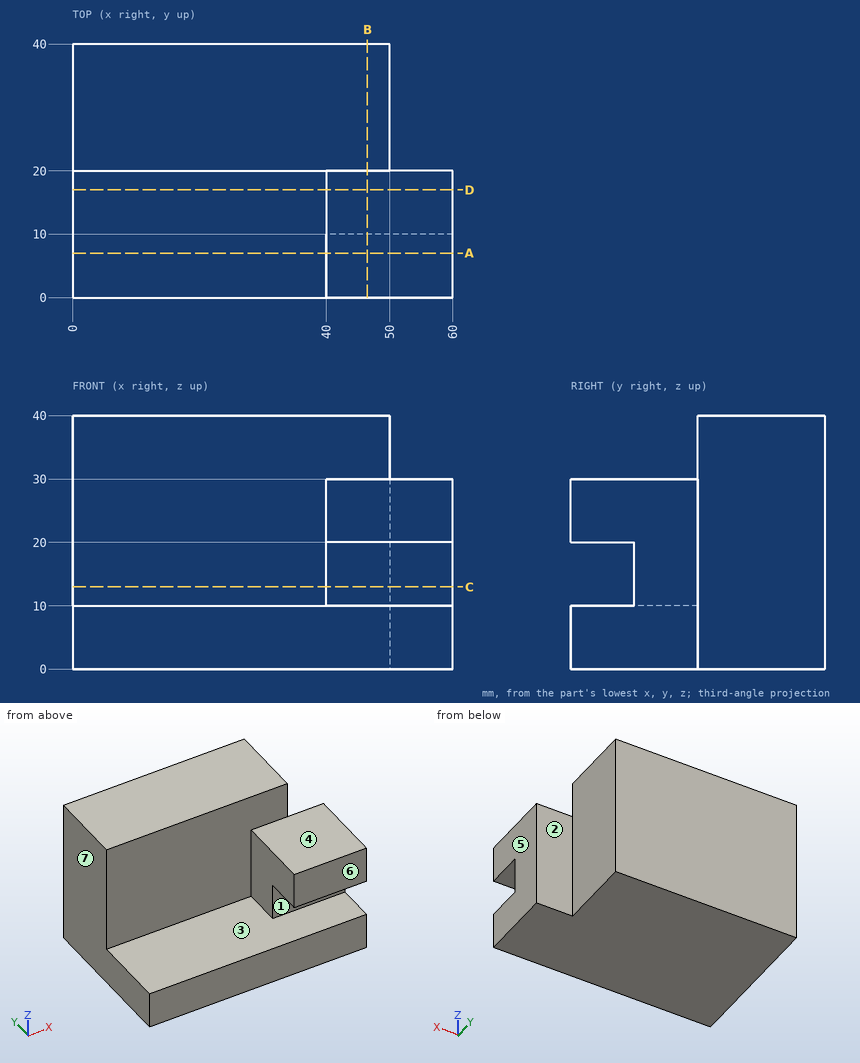
Drawing for the job (mm, zero at the part's lowest x, y, z). A direction names the side the tool comes from. Round coordinates to 2 decimals unless told otherwise and drop trailing zeros. Order: outer loops, then holes, each group sorted by start corner. A loop starts at its lowest first (then second) coordinate and runs counter-clockwise, first axis right, second up.
Item 1: Saw through at D-D on y = 17. Write the cut outline in (x, z), then the cut area to 3 significant figures.
Item 2: Saw through at B-B on x = 46.5. Write the cut outline in (y, z), then the cut area to 3 significant figures.
Item 3: Mould opens along X. For the marked faces 5, 6 and 7 say: pulls with the +X half, pulls with the -X half, needs draft (parallel to the pull), parting line crosses it, or undercut.
Item 4: Saw through at C-C on z = 13. Write the cut outline in (x, y), then the cut area to 3 significant figures.
Item 5: Pin check, flat tips, straight feed: pin 1 (5 mm diameter, centred on x = 47.5, y = 4.5, fed in from -Z); pin 2 (3 mm diameter, centred on x = 54, z = 18.5, fed in from +Y); pin 3 (6 mm diameter, centred on x = 15.5, y = 10, fed in from +Z); pin 4 (10 mm diameter, centred on y = 29, z = 17, fed in from +X). Stop position of each tip, or through.
Item 6: Saw through at A-A on y = 7. Write the cut outline in (x, z), then the cut area to 3 significant figures.
Item 7: Probe line 1 along Z through (x, y) = (16.5, 10.5); line 2 along X through (y, z) = (8, 22); line 3 along Y through (x, z) = (15.5, 14.5). List the from-to ranges inside material, lowest first.
Item 8: Tool access for the marked faces 1, 2, 3 and 4: list every direction of +Z, -Z, +X, -X, +Y, -Y with a clear straight run to the whole face (end or side of a thin tool).
Reported:
1. outline: (0, 0) - (60, 0) - (60, 30) - (40, 30) - (40, 10) - (0, 10) - close
1. area: 1,000 mm2
2. outline: (0, 0) - (40, 0) - (40, 40) - (20, 40) - (20, 30) - (0, 30) - (0, 20) - (10, 20) - (10, 10) - (0, 10) - close
2. area: 1,300 mm2
3. face 5: pulls with the +X half
3. face 6: needs draft
3. face 7: pulls with the -X half
4. outline: (0, 20) - (40, 20) - (40, 10) - (60, 10) - (60, 20) - (50, 20) - (50, 40) - (0, 40) - close
4. area: 1,200 mm2
5. pin 1: stops at z = 0
5. pin 2: stops at y = 20
5. pin 3: stops at z = 10
5. pin 4: stops at x = 50
6. outline: (0, 0) - (60, 0) - (60, 10) - (0, 10) - close; (40, 20) - (60, 20) - (60, 30) - (40, 30) - close
6. area: 800 mm2
7. line 1: z = 0 to 10
7. line 2: x = 40 to 60
7. line 3: y = 20 to 40
8. face 1: +X, -X, -Y
8. face 2: +Z, -Z, +X, +Y
8. face 3: -X, -Y
8. face 4: +Z, +X, -X, -Y
